Verification items for the finished model (mm, model axes). Coordinates: 2 decimals unless noted, no trailing zeros. Order: outer loops, then holes, each group sorted by start corner. A loop starts at its lowest first (then second) coordinate and runs counter-clockwise, first axis right, second up.
Q1. Cross-section at C-C, the plane y = -3. Count the separate pieces of the cut face and the enclosed holes in it, and give its area (3 significant figures).
Q2. Thickness scan on line 1 (Z direction, x = -68.5, y = -2.75); line 2 (Z direction, x = -19.05, y = -1.5); line 3 (X direction, y = -1.75, z = 330.2). Record the ranges inside material, lowest first.
Q3. Cross-section at B-B, the plane x = -60. Record the boundary of the cut face in (y, z), and give its area (3 significant figures).
Q4. Cross-section at D-D, the plane x = -77. Record the boundary of the cut face in (y, z).
Q5. Depth check by flat-ended pin: P1, Ø6.5, axis at x = -94.34, z = 225.42, coming from the -Y side; P2, Ø1, axis at y = -2.5, z = 255, coming from the -X side; P3, Ø1.5, axis at y = -5, z = 196.5, coming from the -X side. Enter the tip coordinate at first touch or a pass-through.
Q6. Cross-section at A-A, the plane z = 101.6. Record the boundary of the cut face in (x, y).
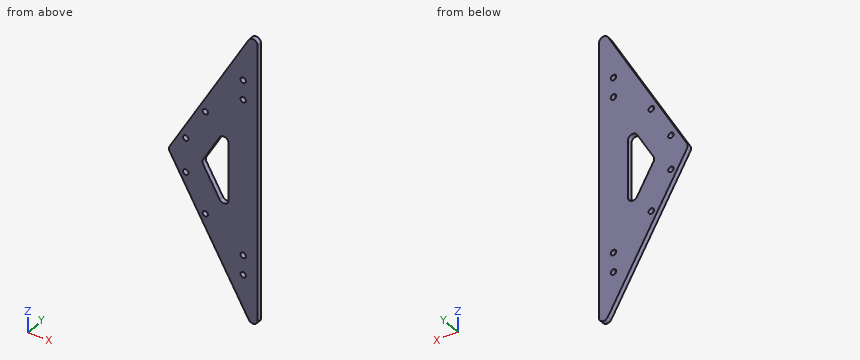
from build123d import *

# Parameters (mm, degrees)
F1_DEPTH = 6.35
F3_D     = 7.1374
F3_DEPTH = 304.8
F3_TIP   = 2.1442912911


# Not quite as in the source:
# - a feature names something its author has since deleted; it is built from what else it names


with BuildPart() as f1:
    # F0 (on Front) → F1 (new body)
    with BuildSketch(Plane.XZ):
        with BuildLine():
            ThreePointArc((-11.849261314, 20.5235226281), (-4.7064990636, 17.5648936311), (0, 23.6985226281))
            Line((0, 23.6985226281), (0, 382.7014773719))
            ThreePointArc((0, 382.7014773719), (-4.7064990636, 388.8351063689), (-11.849261314, 385.8764773719))
            Line((-11.849261314, 385.8764773719), (-115.4844875947, 206.375))
            ThreePointArc((-115.4844875947, 206.375), (-116.3352262806, 203.2), (-115.4844875947, 200.025))
            Line((-115.4844875947, 200.025), (-11.849261314, 20.5235226281))
        make_face()
        with BuildLine():
            ThreePointArc((-49.949261314, 243.6853416036), (-42.8064990636, 246.6439706005), (-38.1, 240.5103416036))
            Line((-38.1, 240.5103416036), (-38.1, 165.8896583964))
            ThreePointArc((-38.1, 165.8896583964), (-42.8064990636, 159.7560293995), (-49.949261314, 162.7146583964))
            Line((-49.949261314, 162.7146583964), (-71.4903970824, 200.025))
            ThreePointArc((-71.4903970824, 200.025), (-72.3411357684, 203.2), (-71.4903970824, 206.375))
            Line((-71.4903970824, 206.375), (-49.949261314, 243.6853416036))
        make_face(mode=Mode.SUBTRACT)
    extrude(amount=F1_DEPTH)

    # F3
    with Locations(Plane.XZ.offset(6.35)):
        with Locations((-94.3381810245, 225.425), (-94.3381810245, 180.975), (-19.05, 304.8), (-19.05, 101.6), (-19.05, 76.2), (-19.05, 330.2), (-68.674961559, 269.875), (-68.674961559, 136.525)):
            Hole(F3_D / 2, depth=F3_DEPTH)
            with Locations((0, 0, -(F3_DEPTH + F3_TIP / 2))):  # 118° drill point
                Cone(0, F3_D / 2, F3_TIP, mode=Mode.SUBTRACT)


solid = f1.part
Check values:
1. separate pieces: 1
1. enclosed holes: 9
1. area: 21,400 mm2
2. line 1: z = 118.65 to 132.96, 140.09 to 194.85, 211.55 to 266.31, 273.44 to 287.75
2. line 2: z = 33 to 72.63, 79.77 to 98.03, 105.17 to 301.23, 308.37 to 326.63, 333.77 to 373.4
2. line 3: x = -43.99 to -22.62, -15.48 to 0
3. outline: (-6.35, 103.92) - (0, 103.92) - (0, 180.12) - (-6.35, 180.12) - close; (-6.35, 226.28) - (0, 226.28) - (0, 302.48) - (-6.35, 302.48) - close
3. area: 968 mm2
4. outline: (-6.35, 133.37) - (0, 133.37) - (0, 273.03) - (-6.35, 273.03) - close
5. P1: passes through
5. P2: stops at x = -87.7
5. P3: stops at x = -113.88
6. outline: (-58.66, -6.35) - (-22.62, -6.35) - (-22.62, 0) - (-58.66, 0) - close; (-15.48, -6.35) - (0, -6.35) - (0, 0) - (-15.48, 0) - close
